```python
from build123d import *

# Parameters (mm, degrees)
F3_DEPTH = 8
F4_W     = 5
F4_H     = 80


with BuildPart() as f1:
    # F0 (on Front) → F1 (revolve)
    with BuildSketch(Plane.XZ):
        Polygon((4, 0), (4, 90), (0, 90), (0, 65), (0, 0), align=None)
    revolve(axis=Axis((0, 0, 32.5), (0, 0, -1)))

    # F2 (on face) → F3 (join)
    with BuildSketch(Plane.XY.offset(90)):
        Polygon((6.968457, -0.663784), (4.059082, 5.702969), (-2.909374, 6.366753), (-6.968457, 0.663784), (-4.059082, -5.702969), (2.909374, -6.366753), align=None)
    extrude(amount=F3_DEPTH)

    # F4 (on Front) → F5 (revolve, cut)
    with BuildSketch(Plane.XZ):
        with Locations((2.5, 40)):
            Rectangle(F4_W, F4_H)
    revolve(axis=Axis((0, 0, 40), (0, 0, -1)), mode=Mode.SUBTRACT)


solid = f1.part
```
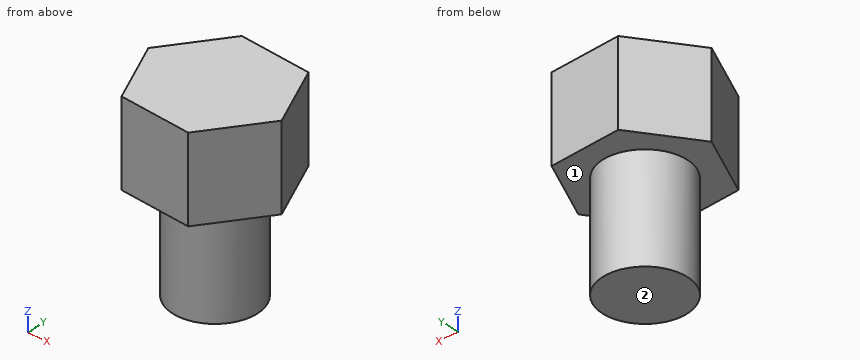
Source: CAD feature listing. Evaluate the final solid. Frame: model axes, mm. Face numbers are marked on the shaded views. A direction names the side the tool comes from. Round coordinates to 2 decimals unless told otherwise and drop trailing zeros. Loops run counter-clockwise (first coordinate to the right, second up) from the corner with the lowest first, then second, coordinate; pieces in that order, holes last. Notation, with made-up numbers: M -3.75,73 L 12.25,73 A14 ccw 12.25,89 Z; hole C 75,-36 d5. An arc over 180 degrees is marked long. Use a Markdown table: item, result. Add a question column.
1. Line query: line 1 (Z direction, x = -3.5, y = 4.5); line 2 (Y direction, x = 2.75, z = 92.5); line 3 (X direction, y = -1.75, z = 84.25). Output: solid intervals per line, ascending.
2. Reachability of the marked faces 1 and 2 from +Z, -Z, +X, -X, +Y, -Y: full face, straight path, thin tool, end or side. Return the list, or none.
3. Contact query for flat-ended pins moving along their axis: P1, Ø2, axis at y = -0.5, z = 95, coming from the -X side; P2, Ø8, axis at x = 1.5, z = 91, coming from the +Y side; P3, Ø2, axis at y = -2.5, z = 95.5, coming from the -X side. Output: stop coordinate, or through.
4. Section query B-B on y = 1.5. Return the cut outline in (x, z), then the cut area to 3 significant figures.
5. Section query A-A on x = -1.25. Return the cut outline in (y, z).
6. Section query C-C on z = 87. Return the cut outline in (x, y).
Reported:
| question | item | result |
|---|---|---|
| 1 | line 1 | z = 90 to 98 |
| 1 | line 2 | y = -6.35 to 5.83 |
| 1 | line 3 | x = -3.6 to 3.6 |
| 2 | face 1 | -Z |
| 2 | face 2 | -Z, +X, -X, +Y, -Y |
| 3 | P1 | stops at x = -6.89 |
| 3 | P2 | stops at y = 6.33 |
| 3 | P3 | stops at x = -5.98 |
| 4 | outline | M -6.37,90 L -3.71,90 L -3.71,80 L 3.71,80 L 3.71,90 L 5.98,90 L 5.98,98 L -6.37,98 Z |
| 4 | area | 173 mm² |
| 5 | outline | M -5.97,90 L -3.8,90 L -3.8,80 L 3.8,80 L 3.8,90 L 6.21,90 L 6.21,98 L -5.97,98 Z |
| 6 | outline | C 0,0 d8 |
